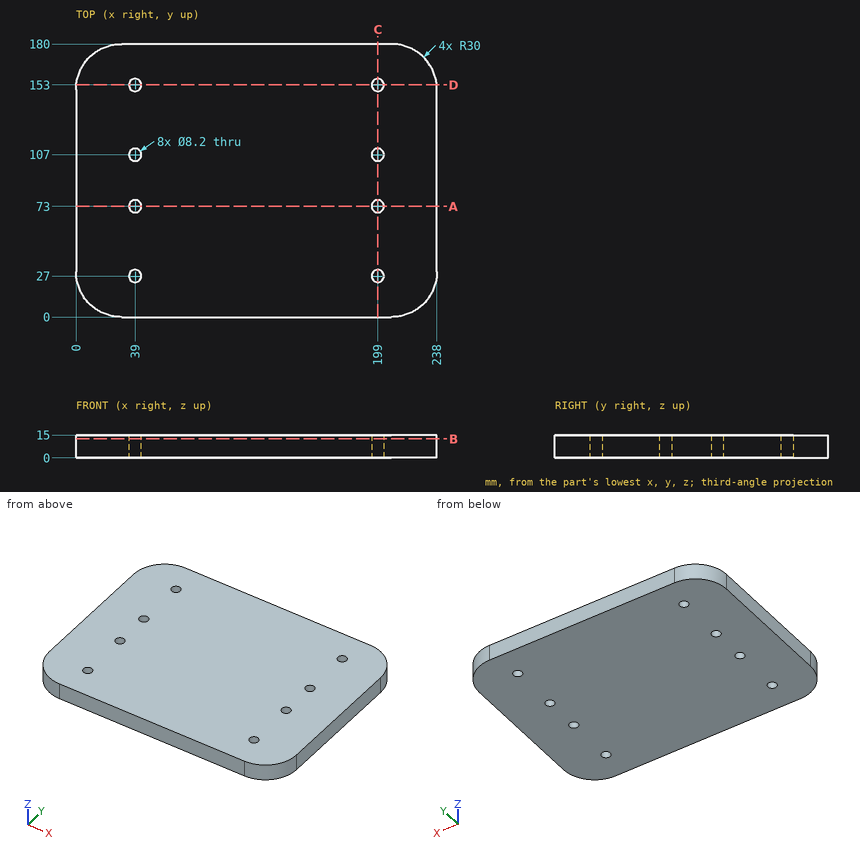
Source: three-view drawing plus pictorial views. Frame: mm from the lowest corner of the part. Give positions to 0.01 mm unless a question says otherwise; leave off trailing zeros. Loops run counter-clockwise (first coordinate to the right, second up) from the corner with the lowest first, then second, coordinate; pieces in that order, holes last. Notation, with made-up numbers: M 52,50.5 L 106,50.5 A14 cw 106,69.5 Z; hole C -1.75,-24.75 d8. An arc over 180 degrees is marked long. Put each result on its own line as item: value.
Q1. Section B-B (z = 12.5). Count the separate pieces of the cut face and the enclosed holes in it, and give its area (3 significant figures).
Response values:
separate pieces: 1
enclosed holes: 8
area: 41,600 mm²
Q2. Section A-A (y = 73). Return the cut outline in (x, z).
Response values:
outline: M 0,0 L 34.9,0 L 34.9,15 L 0,15 Z; M 43.1,0 L 194.9,0 L 194.9,15 L 43.1,15 Z; M 203.1,0 L 238,0 L 238,15 L 203.1,15 Z
Q3. Pin query (flat end, axial travel): P1, Ø6.5, axis at x = 199, y = 107, coming from the +Z side; P2, Ø8, axis at y = 19, z = 11, coming from the -X side. Return the tip coordinate at first contact, or that it passes through.
Response values:
P1: passes through
P2: stops at x = 0.83
Q4. Section C-C (x = 199). Return the cut outline in (y, z).
Response values:
outline: M 0,0 L 22.9,0 L 22.9,15 L 0,15 Z; M 31.1,0 L 68.9,0 L 68.9,15 L 31.1,15 Z; M 77.1,0 L 102.9,0 L 102.9,15 L 77.1,15 Z; M 111.1,0 L 148.9,0 L 148.9,15 L 111.1,15 Z; M 157.1,0 L 180,0 L 180,15 L 157.1,15 Z
Q5. Section D-D (y = 153). Return the cut outline in (x, z), and give its area (3 significant figures).
Response values:
outline: M 0.15,0 L 34.9,0 L 34.9,15 L 0.15,15 Z; M 43.1,0 L 194.9,0 L 194.9,15 L 43.1,15 Z; M 203.1,0 L 237.85,0 L 237.85,15 L 203.1,15 Z
area: 3,320 mm²
Q6. Line query: probe 1 along Y at (x, z) = (199, 9); probe 2 along X at (y, z) = (107.5, 3); probe 3 along X at (y, z) = (152.5, 12.75). Output: solid intervals per line, ascending. Write a range as [from, to].
Response values:
probe 1: y = [0, 22.9], [31.1, 68.9], [77.1, 102.9], [111.1, 148.9], [157.1, 180]
probe 2: x = [0, 34.93], [43.07, 194.93], [203.07, 238]
probe 3: x = [0.1, 34.93], [43.07, 194.93], [203.07, 237.9]
